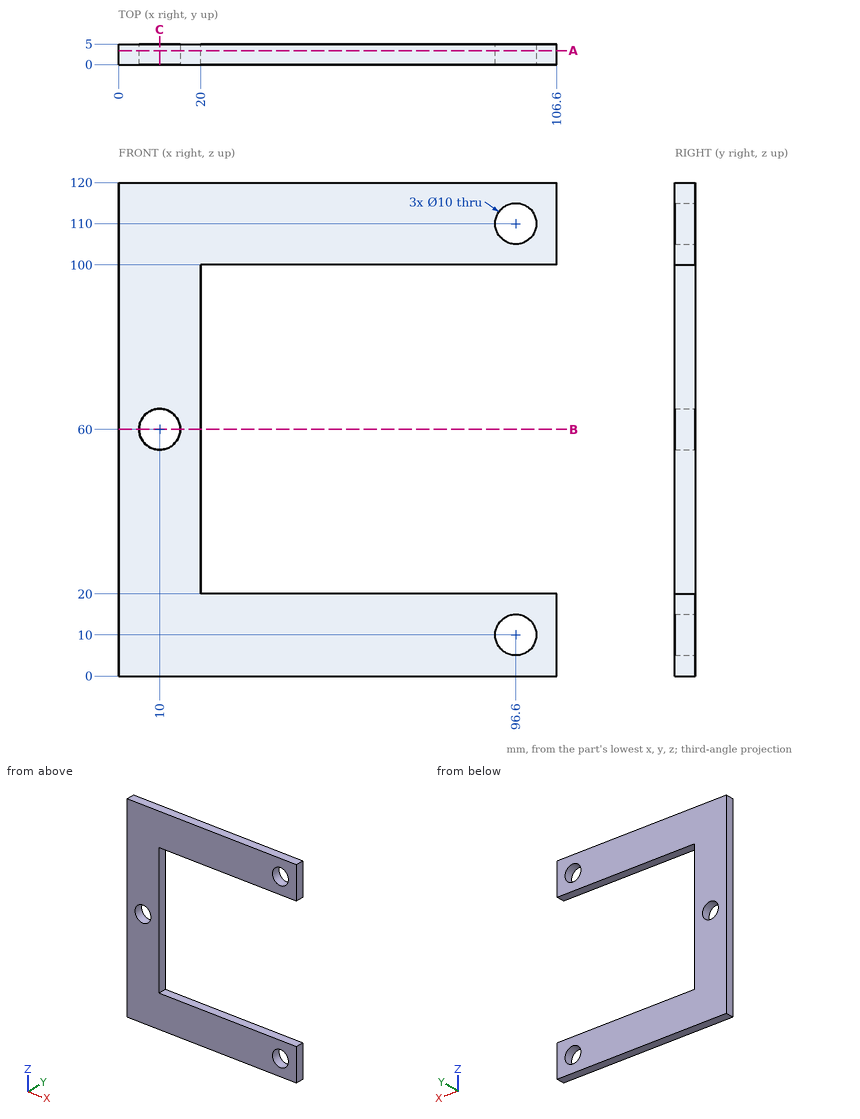
Study the drawing (mm; zero at the part's minimum x, y, z) and answer. Round coordinates to 2 decimals unless told otherwise and drop trailing zeros. Write each loop counter-clockwise with the first axis right and the second up, starting at its lowest first coordinate (ties: lowest second). Pieces come first, ordered by that corner, then holes. Notation, with made-up numbers: (25, 84.25) - (75, 84.25) arc R16 ccw to (75, 108.25) - close; hole circle Ø10 at (18.5, -3). An arc over 180 degrees is marked (long way). Return JSON: item names as keys, results as strings. Group by question number.
Q1. The part is cut by section C-C on x = 10. Write down the section's boundary in (y, z), then the cut area to 3 significant figures.
Q2. Find the intervals of material crossed by L1, parallel to Z at x = 96.6, y = 3.4; L2, parallel to Z at x = 10, y = 4.05; L3, parallel to Z at x = 47.5, y = 4.65, in increasing order.
Q3. The part is cut by section B-B on z = 60. Write down the section's boundary in (x, y), then the cut area to 3 significant figures.
Q4. The part is cut by section A-A on y = 3.4. Write down the section's boundary in (x, z).
Q5. Each of these flat-tipped pins is pushed along its axis until it touches: pin 1 Ø1.5 at (y, z) = (1.5, 79.5) entering from +X; pin 2 Ø9 at (x, z) = (96.6, 110) entering from -Y. Where does it stop, or does it pass through?
Solved:
{
 "1": {"outline": "(0, 0) - (5, 0) - (5, 55) - (0, 55) - close; (0, 65) - (5, 65) - (5, 120) - (0, 120) - close", "area": "550 mm²"},
 "2": {"L1": "0 to 5, 15 to 20, 100 to 105, 115 to 120", "L2": "0 to 55, 65 to 120", "L3": "0 to 20, 100 to 120"},
 "3": {"outline": "(0, 0) - (5, 0) - (5, 5) - (0, 5) - close; (15, 0) - (20, 0) - (20, 5) - (15, 5) - close", "area": "50.0 mm²"},
 "4": {"outline": "(0, 0) - (106.6, 0) - (106.6, 20) - (20, 20) - (20, 100) - (106.6, 100) - (106.6, 120) - (0, 120) - close; hole circle Ø10 at (10, 60); hole circle Ø10 at (96.6, 10); hole circle Ø10 at (96.6, 110)"},
 "5": {"pin 1": "x = 20", "pin 2": "through"}
}
